The listing builds one solid part. Answer for the finished solid, in the listing's coordinates (mm). Face numbers are marked on the shaded views. A direction names the side the tool comes from. Give positions to 0.01 mm unless a question says otherwise; leave off trailing zeros. Write each loop counter-clockwise with the first axis right and the second up, starting at its lowest first coordinate (ties: lowest second). Pieces come first, ordered by that corner, then holes. Notation, with made-up numbers: (61.25, 29.5) - (95.25, 29.5) arc R15 cw to (95.25, 46.5) - close; hole circle Ø8 at (-11, -35). An arc over 180 degrees is marked (long way). Return JSON: item names as keys, results as strings.
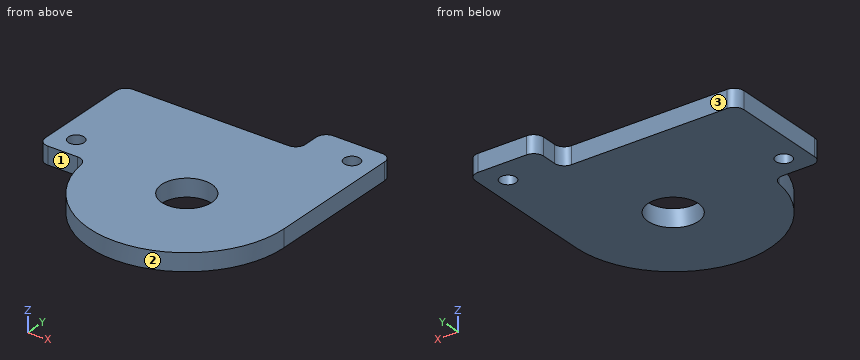
Autodesk Inventor part; units mm, degrees
ref_plane "YZ Plane" through (0, 0, 0) normal (1, 0, 0) x (0, 1, 0)
ref_plane "XZ Plane" through (0, 0, 0) normal (0, 1, 0) x (-1, 0, 0)
ref_plane "XY Plane" through (0, 0, 0) normal (0, 0, 1) x (1, 0, 0)
sketch "Sketch1" plane through (0, 0, 0) normal (0, 0, 1) x (1, 0, 0)
  circle A0 centre (24.9974, -44.3363) radius 20
  line L0 (44.9974, -44.3363) -> (30.9974, -44.3363)
  line L1 (30.9974, -44.3363) -> (30.9974, -14.3363)
  line L2 (30.9974, -14.3363) -> (44.9974, -14.3363)
  line L3 (44.9974, -14.3363) -> (44.9974, -44.3363)
  line L4 (30.9974, -21.407) -> (-4.9442, -21.407)
  line L5 (-4.9442, -21.407) -> (-4.9442, -45.1154)
  line L6 (-4.9442, -45.1154) -> (30.9974, -45.1154)
  line L7 (30.9974, -45.1154) -> (30.9974, -21.407)
  point P0 (0, 0)
  dimension "d0" = 40
  dimension "d1" = 14
  dimension "d2" = 30
extrude "Extrusion1" add sketch "Sketch1" along normal blind 3.6
sketch "Sketch2" plane through (0, 0, 3.6) normal (0, 0, 1) x (1, 0, 0)
  arc A0 (5.0125, -45.1154) -> (44.9974, -44.3363) centre (24.9974, -44.3363) ccw
  circle A1 centre (24.9974, -44.3363) radius 5.15
  circle A2 centre (-0.4442, -40.6154) radius 1.625
  line L0 (-4.9442, -21.407) -> (-4.9442, -45.1154)
  line L1 (-4.9442, -45.1154) -> (5.0125, -45.1154)
  circle A3 centre (40.4974, -19.3363) radius 1.625
  line L2 (44.9974, -44.3363) -> (44.9974, -14.3363)
  point P0 (0, 0)
  dimension "d5" = 10.3
  dimension "d6" = 3.25
  dimension "d9" = 4.5
  dimension "d10" = 4.5
  dimension "d11" = 3.25
  dimension "d12" = 4.5
  dimension "d13" = 25
extrude "Extrusion2" cut sketch "Sketch2" against normal blind 20
fillet "Fillet1" radius 2 6 edges at (44.9974, -14.3363, 1.8) (-4.9442, -45.1154, 1.8) (30.9974, -14.3363, 1.8) (-4.9442, -21.407, 1.8) (30.9974, -21.407, 1.8) (5.0125, -45.1154, 1.8)
properties part number "p6"
Item 1: A cutting plane is placed at B-B on y = -40. Determine the outline of the cut face in (x, z), then the cut area to 3 significant figures.
Answer below:
{"outline": "(-4.94, 0) - (-1.95, 0) - (-1.95, 3.6) - (-4.94, 3.6) - close; (1.06, 0) - (22.22, 0) - (22.22, 3.6) - (1.06, 3.6) - close; (27.78, 0) - (45, 0) - (45, 3.6) - (27.78, 3.6) - close", "area": "149 mm²"}
Item 2: A cutting plane is placed at A-A on x = 24.5. Determine the outline of the cut face in (y, z).
Answer below:
{"outline": "(-64.33, 0) - (-49.46, 0) - (-49.46, 3.6) - (-64.33, 3.6) - close; (-39.21, 0) - (-21.41, 0) - (-21.41, 3.6) - (-39.21, 3.6) - close"}
Item 3: A cutting plane is placed at C-C on y = -20. Determine the outline of the cut face in (x, z).
Answer below:
{"outline": "(30.91, 0) - (39.01, 0) - (39.01, 3.6) - (30.91, 3.6) - close; (41.98, 0) - (45, 0) - (45, 3.6) - (41.98, 3.6) - close"}
Item 4: A flat-ended cylindrical pin translates along its axis: P1, Ø1.8, axis at x = 18.5, z = 2, coming from the +Y side. Find the tip coordinate at first contact, or state that the pin passes through.
Answer below:
{"P1": "stops at y = -21.41"}
Item 5: Consider L1, parallel to Y at x = -1.5, z = 0.8; L2, parallel to X at y = -18, z = 1.2; L3, parallel to Y at x = -1, z = 0.9. Determine where each line is inside the solid, lowest interval first.
Answer below:
{"L1": "y = -45.12 to -41.85, -39.38 to -21.41", "L2": "x = 31 to 39.57, 41.42 to 45", "L3": "y = -45.12 to -42.14, -39.09 to -21.41"}
Item 6: A cutting plane is placed at D-D on z = 2.1. Determine the outline of the cut face in (x, y) (3 decimals), then the cut area to 3 significant figures.
Answer below:
{"outline": "(-4.944, -43.115) arc R2 ccw to (-2.944, -45.115) - (3.174, -45.115) arc R2 cw to (5.158, -46.863) arc R20 ccw to (44.997, -44.336) - (44.997, -16.336) arc R2 ccw to (42.997, -14.336) - (32.997, -14.336) arc R2 ccw to (30.997, -16.336) - (30.997, -19.407) arc R2 cw to (28.997, -21.407) - (-2.944, -21.407) arc R2 ccw to (-4.944, -23.407) - close; hole circle Ø3.25 at (-0.444, -40.615); hole circle Ø10.3 at (24.997, -44.336); hole circle Ø3.25 at (40.497, -19.336)", "area": "1,780 mm²"}
Item 7: For the marked faces 1, 2 and 3, determine the directions among +Z, -Z, +X, -X, +Y, -Y from which every point of the face is accessible in a straight line to the end or side of a thin tool.
Answer below:
{"face 1": "+Z, -Z, -X, -Y", "face 2": "+Z, -Z, -Y", "face 3": "+Z, -Z, -X, +Y"}
